```python
from build123d import *

# Parameters (mm, degrees)
SKETCH1_W                  = 93.116399905
SKETCH1_H                  = 11.836399908
BOSS_EXTRUDE1_DEPTH        = 1.6002
BOSS_EXTRUDE2_DEPTH        = 1.6002
CHAMFER1_SIZE              = 2.54
F_2_6_2_6_DIAMETER_HOLE1_D = 2.6
CUT_EXTRUDE1_DEPTH         = 2.6002


with BuildPart() as part:
    # Sketch1 → Boss-Extrude1 (new body)
    with BuildSketch(Plane.XY.offset(1.63)):
        with Locations((-40.639999999, 0)):
            Rectangle(SKETCH1_W, SKETCH1_H)
    extrude(amount=BOSS_EXTRUDE1_DEPTH)

    # Sketch4 → Boss-Extrude2 (add, through all)
    with BuildSketch(Plane(origin=(0, 0, 1.63), x_dir=(-1, 0, 0), z_dir=(0, 0, -1))):
        Polygon((87.198199951, -5.918199954), (69.803821783, -21.189450144), (57.785000156, -21.189450144), (57.785000156, -5.918199954), align=None)
        Polygon((-5.918199954, -5.918199954), (23.494999841, -5.918199954), (23.494999841, -21.189450144), (11.476178214, -21.189450144), align=None)
    extrude(amount=-BOSS_EXTRUDE2_DEPTH)

    # Chamfer1
    chamfer1_edges = [part.edges().sort_by_distance(p)[0] for p in [
        (-57.785000156, -5.918199954, 2.4301),
        (-23.494999841, -5.918199954, 2.4301),
    ]]
    chamfer(chamfer1_edges, length=CHAMFER1_SIZE)

    # Ø2.6 (2.6) Diameter Hole1 (through all)
    with Locations(Plane.XY.offset(3.2302)):
        with Locations((-10.160000092, -7.6e-08), (-71.119999812, -3.5e-08), (-77.798317195, -12.855075132), (-3.481682742, -12.855075132)):
            Hole(F_2_6_2_6_DIAMETER_HOLE1_D / 2)

    # Sketch6 → Cut-Extrude1 (cut, through all)
    with BuildSketch(Plane(origin=(0, 0, 1.63), x_dir=(-1, 0, 0), z_dir=(0, 0, -1))):
        Polygon((79.427543726, -12.740383202), (78.775241344, -11.997392669), (76.821393045, -13.712757594), (77.473695428, -14.455748127), align=None)
        Polygon((1.852456271, -12.740383202), (3.806304569, -14.455748127), (4.458606952, -13.712757594), (2.504758653, -11.997392669), align=None)
    extrude(amount=-CUT_EXTRUDE1_DEPTH, mode=Mode.SUBTRACT)


solid = part.part
```
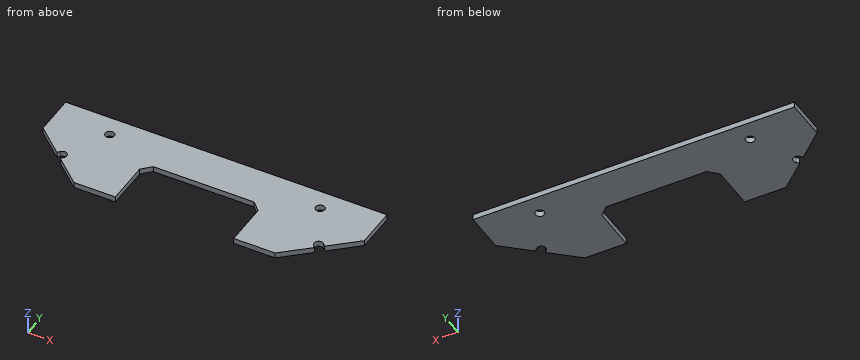
For this review, take the finished solid that the model builds, in its own axes (mm). Coordinates: 2 decimals unless noted, no trailing zeros. Order: outer loops, then holes, each group sorted by start corner. A loop starts at its lowest first (then second) coordinate and runs counter-clockwise, first axis right, second up. Notation, with made-up numbers: (43.25, 3) - (74.25, 3) arc R19 cw to (74.25, 21) - close; hole circle Ø4 at (22.5, 4). An arc over 180 degrees is marked (long way). Answer as a JSON object with one key per item and string values. Group by question number.
1. We need section B-B on y = 0. State the section outline as (x, z) points.
2. We need section C-C on x = -71.5. State the section outline as (y, z) points.
3. We need section A-A on z = 2.8. State the section outline as (x, y) points (3 decimals), then the cut area to 3 significant figures.
4. Clearance check with a flat-ended pin moving along its axis: P1, Ø0.8, axis at y = -14, z = 2.5, coming from the +X side. State where the tip first meets the part, or that it passes through.
5. For probe 1 along X at (y, z) = (0, 2.85); probe 2 along X at (y, z) = (-13, 2.8) (3 decimals); probe 3 along Y at (x, z) = (-43, 2.9), list the stretches that pass through material, from the lowest coordinate up.
Final values:
{
 "1": {"outline": "(-87.2, 1.63) - (-72.42, 1.63) - (-72.42, 3.23) - (-87.2, 3.23) - close; (-69.82, 1.63) - (-11.46, 1.63) - (-11.46, 3.23) - (-69.82, 3.23) - close; (-8.86, 1.63) - (5.92, 1.63) - (5.92, 3.23) - (-8.86, 3.23) - close"},
 "2": {"outline": "(-19.7, 1.63) - (-1.24, 1.63) - (-1.24, 3.23) - (-19.7, 3.23) - close; (1.24, 1.63) - (5.92, 1.63) - (5.92, 3.23) - (1.24, 3.23) - close"},
 "3": {"outline": "(-87.198, -5.918) - (-79.428, -12.74) - (-78.775, -11.997) arc R1.3 cw to (-76.821, -13.713) - (-77.474, -14.456) - (-69.804, -21.189) - (-57.785, -21.189) - (-57.785, -8.458) - (-55.245, -5.918) - (-26.035, -5.918) - (-23.495, -8.458) - (-23.495, -21.189) - (-11.476, -21.189) - (-3.806, -14.456) - (-4.459, -13.713) arc R1.3 cw to (-2.505, -11.997) - (-1.852, -12.74) - (5.918, -5.918) - (5.918, 5.918) - (-87.198, 5.918) - close; hole circle Ø2.6 at (-71.12, 0); hole circle Ø2.6 at (-10.16, 0)", "area": "1,720 mm²"},
 "4": {"P1": "x = -3.86"},
 "5": {"probe 1": "-87.2 to -72.42, -69.82 to -11.46, -8.86 to 5.92", "probe 2": "-76.506 to -57.785, -23.495 to -4.774", "probe 3": "-5.92 to 5.92"}
}
